Part model, mm, in its own coordinate system. Give positions to 0.01 mm unless a question says otherwise; leave off trailing zeros. Write each loop counter-clockwise with the first axis right and the second up, starting at its lowest first coordinate (ties: lowest second). Pieces come first, ordered by that corner, then holes. Notation, with made-up numbers: M 73.5,71.5 L 100.5,71.5 A16 cw 100.5,78.5 Z; hole C 9.25,0 d11. An arc over 180 degrees is marked long. Use CSV: the item, a comma, the result in double quotes. Start each with the question number.
1. Drill centre lines: line 1 along Y through (x, z) = (-50, 1.3); line 2 along Y through (x, z) = (90, 1); line 3 along Y through (x, z) = (61, 1.8). Where is each one in solid material? Low to high. Write a range as from..to.
2. Band-saw the part on A-A, the plane x = -19. List the corners of the cut face in (y, z).
3. Band-saw the part on D-D, the plane y = 10.5. List the corners of the cut face in (x, z).
4. Drop flat-ended pins along their axis: pin 1 Ø0.9 at (y, z) = (-19.5, 2) entering from -X; pin 2 Ø1.5 at (x, z) = (-87.5, 1) entering from +Y; pin 3 Ø1.5 at (y, z) = (-62.5, 2.5) entering from +X. Give the stop position or say it passes through.
5. Band-saw the part on C-C, the plane x = -90. List the corners of the cut face in (y, z), then the cut area to 3 significant figures.
6. Band-saw the part on B-B, the plane y = 50. List the corners of the cut face in (x, z).
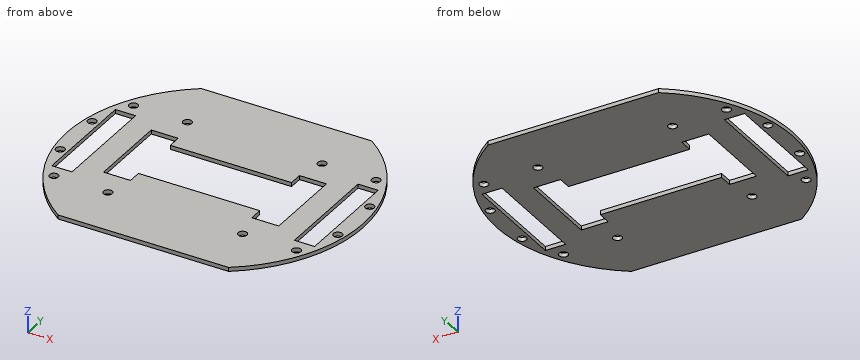
from build123d import *

# Parameters (mm, degrees)
F1_DEPTH = 3
F3_D     = 6.5
F5_D     = 6.5
F6_W     = 90
F6_H     = 40
F7_DEPTH = 3.001
F9_DEPTH = 3.001


# Not quite as in the source:
# - a feature names something its author has since deleted; it is built from what else it names


with BuildPart() as f1:
    # F0 (on Top) → F1 (new body)
    with BuildSketch(Plane.XY):
        with BuildLine():
            Line((63.2455532034, 90), (-63.2455532034, 90))
            ThreePointArc((-63.2455532034, 90), (-110, 0), (-63.2455532034, -90))
            Line((-63.2455532034, -90), (63.2455532034, -90))
            ThreePointArc((63.2455532034, -90), (110, 0), (63.2455532034, 90))
        make_face()
    extrude(amount=F1_DEPTH)

    # F3 (through all)
    with Locations(Plane.XY.offset(3)):
        with Locations((-103, 20), (-103, -20), (-90, 50), (-90, -50), (90, -50), (90, 50), (103, 20), (103, -20)):
            Hole(F3_D / 2)

    # F5 (through all)
    with Locations(Plane.XY.offset(3)):
        with Locations((-50, 50), (50, 50), (50, -50), (-50, -50)):
            Hole(F5_D / 2)

    # F6 (on face) → F7 (cut, through all)
    with BuildSketch(Plane.XY.offset(3)):
        Polygon((-45, -20), (-45, 20), (-45, 30), (-65, 30), (-65, -30), (-45, -30), align=None)
        Rectangle(F6_W, F6_H)
        Polygon((45, 30), (45, 20), (45, -20), (45, -30), (65, -30), (65, 30), align=None)
    extrude(amount=-F7_DEPTH, mode=Mode.SUBTRACT)

    # F8 (on face) → F9 (cut, through all)
    with BuildSketch(Plane.XY.offset(3)):
        Polygon((-90, 40), (-97.5, 40), (-97.5, -40), (-82.5, -40), (-82.5, 40), align=None)
        Polygon((90, 40), (82.5, 40), (82.5, -40), (97.5, -40), (97.5, 40), align=None)
    extrude(amount=-F9_DEPTH, mode=Mode.SUBTRACT)


solid = f1.part
Output:
1,line 1,"y = -90..-53.25, -46.75..-30, 30..46.75, 53.25..90"
1,line 2,"y = -63.25..-53.25, -46.75..-40, 40..46.75, 53.25..63.25"
1,line 3,"y = -90..-30, 30..90"
2,outline,"M -90,0 L -20,0 L -20,3 L -90,3 Z; M 20,0 L 90,0 L 90,3 L 20,3 Z"
3,outline,"M -109.5,0 L -97.5,0 L -97.5,3 L -109.5,3 Z; M -82.5,0 L -65,0 L -65,3 L -82.5,3 Z; M 65,0 L 82.5,0 L 82.5,3 L 65,3 Z; M 97.5,0 L 109.5,0 L 109.5,3 L 97.5,3 Z"
4,pin 1,"stops at x = -108.34"
4,pin 2,"stops at y = 67.63"
4,pin 3,"stops at x = 91.03"
5,outline,"M -63.25,0 L -53.25,0 L -53.25,3 L -63.25,3 Z; M -46.75,0 L -40,0 L -40,3 L -46.75,3 Z; M 40,0 L 46.75,0 L 46.75,3 L 40,3 Z; M 53.25,0 L 63.25,0 L 63.25,3 L 53.25,3 Z"
5,area,"100 mm²"
6,outline,"M -97.98,0 L -93.25,0 L -93.25,3 L -97.98,3 Z; M -86.75,0 L -53.25,0 L -53.25,3 L -86.75,3 Z; M -46.75,0 L 46.75,0 L 46.75,3 L -46.75,3 Z; M 53.25,0 L 86.75,0 L 86.75,3 L 53.25,3 Z; M 93.25,0 L 97.98,0 L 97.98,3 L 93.25,3 Z"
